Geometry check sheet. Reference: the model listing, model coordinates, mm. A direction names the side the tool comes from. Round coordinates to 2 decimals unless told otherwise and drop trailing zeros. Order: outer loops, then holes, each group sorted by start corner. A loop starts at its lowest first (then second) coordinate and runs counter-clockwise, first axis right, second up. Notation, with made-up numbers: (72, 86.25) - (117, 86.25) arc R24 ccw to (117, 108.25) - close; hole circle Ø6 at (-21.5, -4.75). An arc over 180 degrees is marked (long way). Write each question's results on one line, items separated by ' | '.
```python
from build123d import *

# Parameters (mm, degrees)
BOSS_EXTRUDE1_DEPTH = 6
SKETCH2_R           = 8.15711865
CUT_EXTRUDE1_DEPTH  = 10


with BuildPart() as part:
    # Sketch1 → Boss-Extrude1 (new body)
    with BuildSketch(Plane(origin=(0, 0, 0), x_dir=(-1, 0, 0), z_dir=(0, 1, 0))):
        Polygon((-79.827586207, -104.482758621), (-79.827586207, -98.482758621), (134.972413793, -98.482758621), (134.972413793, -104.482758621), (173.972413793, -104.482758621), (173.972413793, -85.022758621), (179.972413793, -85.022758621), (179.972413793, -45.022758621), (173.972413793, -45.022758621), (173.972413793, -20.022758621), (179.972413793, -20.022758621), (179.972413793, 19.977241379), (173.972413793, 19.977241379), (173.972413793, 54.977241379), (179.972413793, 54.977241379), (179.972413793, 95.517241379), (-124.827586207, 95.517241379), (-124.827586207, 54.977241379), (-118.827586207, 54.977241379), (-118.827586207, 19.977241379), (-124.827586207, 19.977241379), (-124.827586207, -20.022758621), (-118.827586207, -20.022758621), (-118.827586207, -45.022758621), (-124.827586207, -45.022758621), (-124.827586207, -85.022758621), (-118.827586207, -85.022758621), (-118.827586207, -104.482758621), align=None)
    extrude(amount=BOSS_EXTRUDE1_DEPTH)

    # Sketch2 → Cut-Extrude1 (cut)
    with BuildSketch(Plane.XZ):
        with Locations(Location((-111.585458186, -66.257055968, 0), (0, 0, 270))):
            Circle(SKETCH2_R)
    extrude(amount=-CUT_EXTRUDE1_DEPTH, mode=Mode.SUBTRACT)


solid = part.part
```
(1) Material ranges on line 1 (Z direction, x = -35.5, y = 4.5); line 2 (X direction, y = 3.3, z = -94.5); line 3 (X direction, y = 0.6, z = -69), recorded low to high.
Answers follow:
line 1: -98.48 to 95.52 | line 2: -173.97 to 118.83 | line 3: -179.97 to -119.27, -103.9 to 124.83
(2) Access from +Z, -Z, +X, -X, +Y, -Y to the whole of each face (thin tool, end or side, straight path). Record for faces 1 (the face through (118.828, 3, -95)), 2 (the face through (-177, 3, 54.977)), 3 (the face through (124.828, 3, -65)), 4 (the face through (122, 3, -45.023)).
Answers follow:
face 1: -Z, +X, +Y, -Y | face 2: -X, +Y, -Y | face 3: +Z, -Z, +X, +Y, -Y | face 4: +X, +Y, -Y
(3) Draft check along X on faces 5 (the face through (-109.14, 2.96, -74.04)), 6 (the face through (-26, 3, -98.483)), 7 (the face through (-177, 3, -20.023)), 8 (the face through (-173.972, 3, 37)). Enter one of: released by +X, released by -X, zero draft, split by the parting line, or undercut.
Answers follow:
face 5: undercut | face 6: undercut | face 7: zero draft | face 8: released by -X
(4) Section check C-C (x = -33.5). Record the cut outline in (y, z).
Answers follow:
outline: (0, -98.48) - (6, -98.48) - (6, 95.52) - (0, 95.52) - close
(5) Section check B-B (z = 39). Record the cut outline in (x, y), then the cut area to 3 significant figures.
Answers follow:
outline: (-173.97, 0) - (118.83, 0) - (118.83, 6) - (-173.97, 6) - close | area: 1,760 mm²
(6) Depth check by flat-ended pin: pin 1 Ø1.8 at (y, z) = (3.5, -96.5) entering from +X; pin 2 Ø1.8 at (y, z) = (3.5, 38) entering from -X; pin 3 Ø1.8 at (x, y) = (-177, 2) entering from -Z. Enter the tip coordinate at first touch or a pass-through.
Answers follow:
pin 1: x = 118.83 | pin 2: x = -173.97 | pin 3: z = -85.02
